For this review, take the finished solid that the model builds, in its own axes (mm). Round coordinates to 2 decimals unless told otherwise and drop trailing zeros. Order: outer loops, then holes, each group sorted by start corner. A loop starts at its lowest first (then second) coordinate and runs counter-clockwise, first axis right, second up. Notation, with made-up numbers: (-37, -10) - (-23, -10) arc R23 cw to (-23, 29) - close; hole circle Ø9 at (35.5, -8). An arc over 180 degrees is marked (long way). One line per question, with ' | ' between items.
```python
from build123d import *

# Parameters (mm, degrees)
SALIENTE_EXTRUIR2_DEPTH = 41.275
CROQUIS2_5_OUTSIDE_W    = 604.615
CROQUIS2_5_OUTSIDE_H    = 671.29
CORTAR_EXTRUIR2_DEPTH   = 41.275
SALIENTE_EXTRUIR4_DEPTH = 2.54
CROQUIS3_5_OUTSIDE_W    = 604.997
CROQUIS3_5_OUTSIDE_H    = 184.309
CROQUIS3_5_OUTSIDE_R    = 1.735738664
CORTAR_EXTRUIR3_DEPTH   = 2.54
REDONDEO1_R             = 12.7
REDONDEO2_R             = 12.7
REDONDEO3_R             = 12.7
REDONDEO4_R             = 12.7
REDONDEO5_R             = 12.7
REDONDEO6_R             = 12.7
REDONDEO7_R             = 12.7
REDONDEO8_R             = 12.7
REDONDEO9_R             = 12.7
REDONDEO10_R            = 12.7
REDONDEO11_R            = 12.7
REDONDEO12_R            = 12.7


with BuildPart() as part:
    # Croquis2 → Saliente-Extruir2 (new body)
    with BuildSketch(Plane(origin=(0, 0, 0), x_dir=(1, 0, 0), z_dir=(0, 1, 0))):
        Polygon((409.380647902, 498.22250712), (409.380647902, -30.41499288), (55.368147902, -30.41499288), (-52.581852098, 37.05375712), (-52.581852098, 430.75375712), (55.368147902, 498.22250712), align=None)
    extrude(amount=SALIENTE_EXTRUIR2_DEPTH)

    # Croquis2<5> outside → Cortar-Extruir2 (cut)
    # profile 1 of 2: a face of its own
    with BuildSketch(Plane(origin=(0, 0, 0), x_dir=(1, 0, 0), z_dir=(0, 1, 0))):
        with Locations((178.3995, 233.904)):
            Rectangle(CROQUIS2_5_OUTSIDE_W, CROQUIS2_5_OUTSIDE_H)
        Polygon((409.380647902, 498.22250712), (409.380647902, -30.41499288), (55.368147902, -30.41499288), (-52.581852098, 37.05375712), (-52.581852098, 430.75375712), (55.368147902, 498.22250712), align=None, mode=Mode.SUBTRACT)
    # profile 2 of 2: a face of its own
    with BuildSketch(Plane(origin=(0, 0, 0), x_dir=(1, 0, 0), z_dir=(0, 1, 0))):
        Polygon((55.368147902, 15.62250712), (372.868147902, 15.62250712), (372.868147902, 452.18500712), (55.368147902, 452.18500712), (-16.069352098, 409.32250712), (-16.069352098, 58.48500712), align=None)
    extrude(amount=CORTAR_EXTRUIR2_DEPTH, mode=Mode.SUBTRACT)

    # Croquis3 → Saliente-Extruir4 (add)
    with BuildSketch(Plane.XY.offset(30.41499288)):
        with BuildLine():
            Line((217.386255897, 24.306608413), (247.362539906, 24.306608413))
            ThreePointArc((247.362539906, 24.306608413), (251.03164832, 20.6375), (247.362539906, 16.968391587))
            Line((247.362539906, 16.968391587), (217.386255897, 16.968391587))
            ThreePointArc((217.386255897, 16.968391587), (213.717147484, 20.6375), (217.386255897, 24.306608413))
        make_face()
    extrude(amount=SALIENTE_EXTRUIR4_DEPTH)

    # Croquis3<5> outside → Cortar-Extruir3 (cut)
    # profile 1 of 4: a face of its own
    with BuildSketch(Plane.XY.offset(30.41499288)):
        with Locations((178.3995, 20.6375)):
            Rectangle(CROQUIS3_5_OUTSIDE_W, CROQUIS3_5_OUTSIDE_H)
        with BuildLine():
            Line((217.386255897, 24.306608413), (247.362539906, 24.306608413))
            ThreePointArc((247.362539906, 24.306608413), (251.03164832, 20.6375), (247.362539906, 16.968391587))
            Line((247.362539906, 16.968391587), (217.386255897, 16.968391587))
            ThreePointArc((217.386255897, 16.968391587), (213.717147484, 20.6375), (217.386255897, 24.306608413))
        make_face(mode=Mode.SUBTRACT)
    # profile 2 of 4: a face of its own
    with BuildSketch(Plane.XY.offset(30.41499288)):
        with Locations((217.386255897, 20.6375)):
            Circle(CROQUIS3_5_OUTSIDE_R)
    # profile 3 of 4: a face of its own
    with BuildSketch(Plane.XY.offset(30.41499288)):
        with Locations((247.362539906, 20.6375)):
            Circle(CROQUIS3_5_OUTSIDE_R)
    # profile 4 of 4: a face of its own
    with BuildSketch(Plane.XY.offset(30.41499288)):
        with BuildLine():
            Line((228.433365542, 22.195071447), (236.315430261, 22.195071447))
            ThreePointArc((236.315430261, 22.195071447), (237.873001708, 20.6375), (236.315430261, 19.079928553))
            Line((236.315430261, 19.079928553), (228.433365542, 19.079928553))
            ThreePointArc((228.433365542, 19.079928553), (226.875794095, 20.6375), (228.433365542, 22.195071447))
        make_face()
    extrude(amount=CORTAR_EXTRUIR3_DEPTH, mode=Mode.SUBTRACT)

    # Redondeo1
    redondeo1_edges = [part.edges().sort_by_distance(p)[0] for p in [
        (372.868147902, 20.6375, -452.18500712),
    ]]
    fillet(redondeo1_edges, radius=REDONDEO1_R)

    # Redondeo2
    redondeo2_edges = [part.edges().sort_by_distance(p)[0] for p in [
        (372.868147902, 20.6375, -15.62250712),
    ]]
    fillet(redondeo2_edges, radius=REDONDEO2_R)

    # Redondeo3
    redondeo3_edges = [part.edges().sort_by_distance(p)[0] for p in [
        (-16.069352098, 20.6375, -409.32250712),
    ]]
    fillet(redondeo3_edges, radius=REDONDEO3_R)

    # Redondeo4
    redondeo4_edges = [part.edges().sort_by_distance(p)[0] for p in [
        (55.368147902, 20.6375, -452.18500712),
    ]]
    fillet(redondeo4_edges, radius=REDONDEO4_R)

    # Redondeo5
    redondeo5_edges = [part.edges().sort_by_distance(p)[0] for p in [
        (55.368147902, 20.6375, -15.62250712),
    ]]
    fillet(redondeo5_edges, radius=REDONDEO5_R)

    # Redondeo6
    redondeo6_edges = [part.edges().sort_by_distance(p)[0] for p in [
        (-16.069352098, 20.6375, -58.48500712),
    ]]
    fillet(redondeo6_edges, radius=REDONDEO6_R)

    # Redondeo7
    redondeo7_edges = [part.edges().sort_by_distance(p)[0] for p in [
        (55.368147902, 20.6375, 30.41499288),
    ]]
    fillet(redondeo7_edges, radius=REDONDEO7_R)

    # Redondeo8
    redondeo8_edges = [part.edges().sort_by_distance(p)[0] for p in [
        (-52.581852098, 20.6375, -37.05375712),
    ]]
    fillet(redondeo8_edges, radius=REDONDEO8_R)

    # Redondeo9
    redondeo9_edges = [part.edges().sort_by_distance(p)[0] for p in [
        (-52.581852098, 20.6375, -430.75375712),
    ]]
    fillet(redondeo9_edges, radius=REDONDEO9_R)

    # Redondeo10
    redondeo10_edges = [part.edges().sort_by_distance(p)[0] for p in [
        (55.368147902, 20.6375, -498.22250712),
    ]]
    fillet(redondeo10_edges, radius=REDONDEO10_R)

    # Redondeo11
    redondeo11_edges = [part.edges().sort_by_distance(p)[0] for p in [
        (409.380647902, 20.6375, 30.41499288),
    ]]
    fillet(redondeo11_edges, radius=REDONDEO11_R)

    # Redondeo12
    redondeo12_edges = [part.edges().sort_by_distance(p)[0] for p in [
        (409.380647902, 20.6375, -498.22250712),
    ]]
    fillet(redondeo12_edges, radius=REDONDEO12_R)


solid = part.part
```
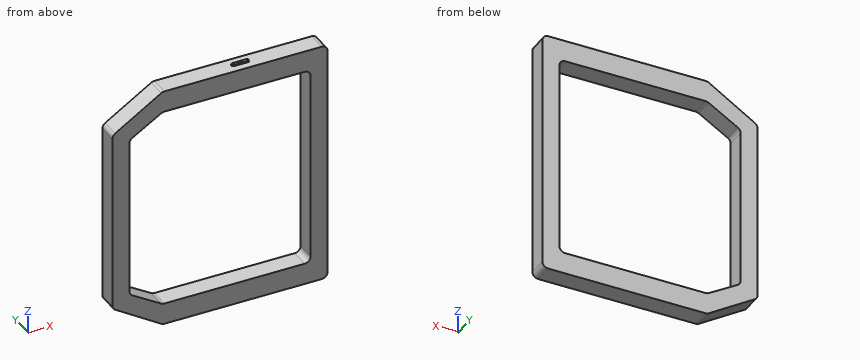
(1) We need section C-C on z = -99.5. State the section outline as (x, y) points (3 decimals), plus the area to 3 significant figures.
Output values:
outline: (-52.582, 0) - (-16.069, 0) - (-16.069, 41.275) - (-52.582, 41.275) - close; (372.868, 0) - (409.381, 0) - (409.381, 41.275) - (372.868, 41.275) - close | area: 3,010 mm^2
(2) Insertion check: pin 1 (8 mm diameter, centred on x = 34.5, y = 30, fed in from +Z); pin 2 (1.3 mm diameter, centred on x = 234, z = 31.5, fed in from -Y); pin 3 (3 mm diameter, centred on y = 23.5, z = -40, fed in from -X). Each pin has a flat end and moves straight along its axis. Give the tip position at first contact, or say it passes through.
Output values:
pin 1: z = 19.87 | pin 2: y = 16.97 | pin 3: x = -52.31
(3) For probe 1 along X at (y, z) = (21, -334); probe 2 along Z at (x, y) = (218, 28) (1 decimal); probe 3 along Z at (x, y) = (29, 20), list the stretches that pass through material, from the lowest coordinate up. Write a range as [from, to].
Output values:
probe 1: [-52.58, -16.07], [372.87, 409.38] | probe 2: [-498.2, -452.2], [-15.6, 30.4] | probe 3: [-481.74, -436.36], [-31.44, 13.93]
(4) We need section A-A on x = 127. State the section outline as (y, z) points (1 decimal), plus the area to 3 significant figures.
Output values:
outline: (0, -498.2) - (41.3, -498.2) - (41.3, -452.2) - (0, -452.2) - close; (0, -15.6) - (41.3, -15.6) - (41.3, 30.4) - (0, 30.4) - close | area: 3,800 mm^2
(5) We need section B-B on y = 9.5. State the section outline as (x, z) points (1 decimal), plus the area to 3 significant figures.
Output values:
outline: (-52.6, -423.7) arc R12.7 ccw to (-46.6, -434.5) - (52.3, -496.3) arc R12.7 ccw to (59, -498.2) - (396.7, -498.2) arc R12.7 ccw to (409.4, -485.5) - (409.4, 17.7) arc R12.7 ccw to (396.7, 30.4) - (59, 30.4) arc R12.7 ccw to (52.3, 28.5) - (-46.6, -33.3) arc R12.7 ccw to (-52.6, -44.1) - close; hole (-16.1, -402.1) arc R12.7 ccw to (-9.9, -413) - (52.4, -450.4) arc R12.7 ccw to (58.9, -452.2) - (360.2, -452.2) arc R12.7 ccw to (372.9, -439.5) - (372.9, -28.3) arc R12.7 ccw to (360.2, -15.6) - (58.9, -15.6) arc R12.7 ccw to (52.4, -17.4) - (-9.9, -54.8) arc R12.7 ccw to (-16.1, -65.7) - close | area: 70,200 mm^2
